```python
from build123d import *

# Parameters (mm, degrees)
BOSS_EXTRUDE3_DEPTH = 10
SKETCH4_R           = 35
SKETCH4_R_2         = 4
BOSS_EXTRUDE4_DEPTH = 10
BOSS_EXTRUDE6_DEPTH = 10
CHAMFER2_SIZE       = 30
CHAMFER2_SIZE2      = 42.426406871
CHAMFER3_SIZE       = 10
CUT_EXTRUDE1_DEPTH  = 20
SKETCH8_R           = 2.5
CUT_EXTRUDE2_DEPTH  = 20
CUT_EXTRUDE4_START  = -10
SKETCH9_R           = 2.5
CUT_EXTRUDE4_DEPTH  = 5
SKETCH10_R          = 11
CUT_EXTRUDE5_DEPTH  = 5


with BuildPart() as part:
    # Sketch3 → Boss-Extrude3 (new body)
    with BuildSketch(Plane(origin=(0, 0, 0), x_dir=(1, 0, 0), z_dir=(0, 1, 0))):
        with BuildLine():
            Line((45, 53.619026474), (35, 53.619026474))
            Line((35, 53.619026474), (35, -53.619026474))
            Line((35, -53.619026474), (45, -53.619026474))
            ThreePointArc((45, -53.619026474), (70, 0), (45, 53.619026474))
        make_face()
    extrude(amount=BOSS_EXTRUDE3_DEPTH)

    # Sketch4 → Boss-Extrude4 (add)
    # profile 1 of 2: a face of its own
    with BuildSketch(Plane.ZY.offset(-35)):
        with BuildLine():
            Line((-53.619026474, 29.121551791), (-53.619026474, 10))
            Line((-53.619026474, 10), (53.619026474, 10))
            Line((53.619026474, 10), (53.619026474, 20.878448209))
            Line((53.619026474, 20.878448209), (-50.251262658, 124.748737342))
            ThreePointArc((-50.251262658, 124.748737342), (-42.664216362, 113.393920133), (-40, 100))
            ThreePointArc((-40, 100), (-61.606079867, 67.664216362), (-99.748737342, 75.251262658))
            Line((-99.748737342, 75.251262658), (-53.619026474, 29.121551791))
        make_face()
    # profile 2 of 2: a face of its own
    with BuildSketch(Plane.ZY.offset(-35)):
        with Locations((-75, 100)):
            Circle(SKETCH4_R)
        with Locations((-75, 100)):
            Circle(SKETCH4_R_2, mode=Mode.SUBTRACT)
    extrude(amount=-BOSS_EXTRUDE4_DEPTH)

    # Sketch6 → Boss-Extrude6 (add)
    with BuildSketch(Plane(origin=(45, 0, 0), x_dir=(0, 0, -1), z_dir=(1, 0, 0))):
        with BuildLine():
            Line((64.393398282, 110.606601718), (-36.213203436, 10))
            Line((-36.213203436, 10), (6.213203436, 10))
            Line((6.213203436, 10), (85.606601718, 89.393398282))
            ThreePointArc((85.606601718, 89.393398282), (85.606601718, 110.606601718), (64.393398282, 110.606601718))
        make_face()
    extrude(amount=BOSS_EXTRUDE6_DEPTH)

    # Chamfer2
    chamfer2_edges = [part.edges().sort_by_distance(p)[0] for p in [
        (50, 10, -6.213203436),
    ]]
    chamfer2_side = [part.faces().sort_by_distance(p)[0] for p in [
        (56.695914019, 10, -4.424051509),
    ]]
    chamfer(chamfer2_edges, length=CHAMFER2_SIZE, length2=CHAMFER2_SIZE2, reference=chamfer2_side[0])

    # Chamfer3
    chamfer3_edges = [part.edges().sort_by_distance(p)[0] for p in [
        (45, 25, -36.213203436),
        (45, 64.696699141, -60.909902577),
        (45, 110.606601718, -85.606601718),
        (45, 60.303300859, -14.090097423),
    ]]
    chamfer(chamfer3_edges, length=CHAMFER3_SIZE - 0.0001)  # a hair under: the kernel refuses the full size

    # Sketch7 → Cut-Extrude1 (cut)
    with BuildSketch(Plane.ZY.offset(-35)):
        with BuildLine():
            Line((18.619026474, 6.380973526), (18.619026474, 0))
            Line((18.619026474, 0), (-18.619026474, 0))
            Line((-18.619026474, 0), (-18.619026474, 31.547958662))
            ThreePointArc((-18.619026474, 31.547958662), (-15.532443636, 36.167356325), (-10.083492568, 35.083492568))
            Line((-10.083492568, 35.083492568), (18.619026474, 6.380973526))
        make_face()
    extrude(amount=-CUT_EXTRUDE1_DEPTH, mode=Mode.SUBTRACT)

    # Sketch8 → Cut-Extrude2 (cut)
    with BuildSketch(Plane.XZ):
        with Locations(Location((45, 31.622776602, 0), (0, 0, 270))):
            Circle(SKETCH8_R)
        with Locations(Location((45, -31.622776602, 0), (0, 0, 270))):
            Circle(SKETCH8_R)
        with Locations(Location((62.5, 0, 0), (0, 0, 270))):
            Circle(SKETCH8_R)
    extrude(amount=-CUT_EXTRUDE2_DEPTH, mode=Mode.SUBTRACT)

    # Sketch9 → Cut-Extrude4 (cut)
    # profile 1 of 4: a face of its own
    with BuildSketch(Plane.XZ.offset(CUT_EXTRUDE4_START)):
        Polygon((55, 26.997776602), (47.670244995, 26.997776602), (50.34048999, 31.622776602), (47.670244995, 36.247776602), (55, 36.213203436), align=None)
    # profile 2 of 4: a face of its own
    with BuildSketch(Plane.XZ.offset(CUT_EXTRUDE4_START)):
        Polygon((42.329755005, 26.997776602), (47.670244995, 26.997776602), (50.34048999, 31.622776602), (47.670244995, 36.247776602), (42.329755005, 36.247776602), (39.65951001, 31.622776602), align=None)
        with Locations(Location((45, 31.622776602, 0), (0, 0, 270))):
            Circle(SKETCH9_R, mode=Mode.SUBTRACT)
    # profile 3 of 4: a face of its own
    with BuildSketch(Plane.XZ.offset(CUT_EXTRUDE4_START)):
        Polygon((55, -36.213203436), (47.670244995, -36.247776602), (50.34048999, -31.622776602), (47.670244995, -26.997776602), (55, -26.997776602), align=None)
    # profile 4 of 4: a face of its own
    with BuildSketch(Plane.XZ.offset(CUT_EXTRUDE4_START)):
        Polygon((42.329755005, -36.247776602), (47.670244995, -36.247776602), (50.34048999, -31.622776602), (47.670244995, -26.997776602), (42.329755005, -26.997776602), (39.65951001, -31.622776602), align=None)
        with Locations(Location((45, -31.622776602, 0), (0, 0, 270))):
            Circle(SKETCH9_R, mode=Mode.SUBTRACT)
    extrude(amount=-CUT_EXTRUDE4_DEPTH, mode=Mode.SUBTRACT)

    # Sketch10 → Cut-Extrude5 (cut)
    with BuildSketch(Plane.ZY.offset(-35)):
        with Locations((-75, 100)):
            Circle(SKETCH10_R)
    extrude(amount=-CUT_EXTRUDE5_DEPTH, mode=Mode.SUBTRACT)


solid = part.part
```
Can you work these out from the model? Positions are in its coordinate system, mm. A direction names the side the tool comes from. Coordinates: 2 decimals unless noted, no trailing zeros. Loops run counter-clockwise (first coordinate to the right, second up) from the corner with the lowest first, then second, coordinate; pieces in that order, holes last. Notation, with made-up numbers: (81, -23) - (101, -23) arc R29 cw to (101, 7) - close; hole circle Ø1 at (-21, 5.25). An arc over 180 degrees is marked (long way). Answer as CSV lines item,"result". Start each with the question number.
1) Suppose I cut it at B-B (x = 62.5). Please give me the cut outline in (y, z), plus the area to 3 significant figures.
2) Which directions (+Z, -Z, +X, -X, +Y, -Y) give clear straight access to the entire face, cutting with the end or side of a thin tool? Please do faces 1 (the flat face through (40, 95, -75)), 2 (the flat face through (40, 15, -53.619)), 3 (the flat face through (45, 91, -29)).
3) I need wall thicknesses on line 1 (X direction, y = 4.5, z = 0); line 2 (X direction, y = 127.5, z = -68.5); line 3 (Z direction, x = 42, y = 25). Which ranges of each line are inside material? Lowest first, please. Write a range as from..to.
4) Thinking about a two-plate mould opening in Y: for faces 4 (the flat face through (49.93, 61.107, -7.723)), 5 (the flat face through (49, 12, 26.998)), 6 (the flat face through (40, 10, 53.619)), which applies, pulls with the +Y half, pulls with the -Y half, needs draft (parallel to the pull), parting line crosses it, or undercut?
5) For pin 1 (4 mm diameter, centred on x = 49, z = -68, fed in from +Y); pin 2 (8 mm diameter, centred on y = 111.5, z = -39.5, fed in from +X); pin 3 (8 mm diameter, centred on x = 42, y = 19, fed in from -Z), each with a flat end and sliding along its axis, tell me the tip position at first contact or that it passes through.
Check result:
1,outline,"(0, -31.52) - (10, -31.52) - (10, -2.5) - (0, -2.5) - close; (0, 2.5) - (10, 2.5) - (10, 31.52) - (0, 31.52) - close"
1,area,"580 mm²"
2,face 1,"-X"
2,face 2,"-Z, +X, -X, -Y"
2,face 3,"+X"
3,line 1,"x = 55..60, 65..70"
3,line 2,"x = 35..45"
3,line 3,"z = -53.62..-18.62, 0..49.5"
4,face 4,"pulls with the +Y half"
4,face 5,"undercut"
4,face 6,"needs draft"
5,pin 1,"stops at y = 122"
5,pin 2,"stops at x = 45"
5,pin 3,"stops at z = -53.62"
